```python
from build123d import *

# Parameters (mm, degrees)
SKETCH1_W           = 33
SKETCH1_H           = 37
BOSS_EXTRUDE1_DEPTH = 33
SKETCH2_R           = 13.75
CUT_EXTRUDE1_DEPTH  = 33
SKETCH3_R           = 3
CUT_EXTRUDE2_DEPTH  = 33


with BuildPart() as part:
    # Sketch1 → Boss-Extrude1 (new body)
    with BuildSketch(Plane.XY):
        with Locations((-16.5, 18.5)):
            Rectangle(SKETCH1_W, SKETCH1_H)
    extrude(amount=BOSS_EXTRUDE1_DEPTH)

    # Sketch2 → Cut-Extrude1 (cut)
    with BuildSketch(Plane.XY.offset(33)):
        with Locations((-16.5, 37)):
            Circle(SKETCH2_R)
    extrude(amount=-CUT_EXTRUDE1_DEPTH, mode=Mode.SUBTRACT)

    # Sketch3 → Cut-Extrude2 (cut)
    with BuildSketch(Plane.ZY.offset(33)):
        with Locations((16.5, 15)):
            Circle(SKETCH3_R)
    extrude(amount=-CUT_EXTRUDE2_DEPTH, mode=Mode.SUBTRACT)


solid = part.part
```
Part model, mm, in its own coordinate system. Round coordinates to 2 decimals unless told otherwise and drop trailing zeros. Order: outer loops, then holes, each group sorted by start corner. A loop starts at its lowest first (then second) coordinate and runs counter-clockwise, first axis right, second up. Notation, with made-up numbers: M 18,73 L 48,73 A17 ccw 48,106 Z; hole C -39.75,11.5 d10. An arc over 180 degrees is marked long. Put each result on its own line as item: value. Start each with the question number.
1. Drill centre lines: probe 1 along X at (y, z) = (25, 16); probe 2 along Y at (x, z) = (-24.5, 16.5); probe 3 along X at (y, z) = (32.5, 28). Where is each one in solid material? Low to high. Write a range as [from, to].
2. Slice it at B-B on y = 31. List the corners of the cut face in (x, z).
3. Drop flat-ended pins along their axis: pin 1 (3.5 mm diameter, centred on y = 15, z = 16.5, fed in from +X); pin 2 (12 mm diameter, centred on x = -18.5, z = 9.5, fed in from +Y); pin 3 (1 mm diameter, centred on x = -28, z = 14.5, fed in from +Y). Give the stop position or say it passes through.
4. Slice it at D-D on z = 10. List the corners of the cut face in (x, y), then the cut area to 3 significant figures.
5. Two-plate mould, pull along Z, no slides. Class faces 1 (the face through (-1, 37, 16)), 2 (the face through (-17, 15, 0)), 3 (the face through (-16.73, 12.07, 15.85)): +Z half, -Z half, draft (parallel to the pull), parting line (faces both ways), or undercut.
6. Slice it at A-A on x = -16.5. List the corners of the cut face in (y, z), then the cut area to 3 significant figures.
7. Slice it at C-C on z = 16.5. List the corners of the cut face in (x, y).
Findings:
1. probe 1: [-33, -23.21], [-9.79, 0]
1. probe 2: [0, 12], [18, 25.82]
1. probe 3: [-33, -29.49], [-3.51, 0]
2. outline: M -33,0 L -28.87,0 L -28.87,33 L -33,33 Z; M -4.13,0 L 0,0 L 0,33 L -4.13,33 Z
3. pin 1: through
3. pin 2: y = 25.82
3. pin 3: y = 30.29
4. outline: M -33,0 L 0,0 L 0,37 L -2.75,37 A13.75 cw -30.25,37 L -33,37 Z
4. area: 924 mm2
5. face 1: draft
5. face 2: -Z half
5. face 3: undercut
6. outline: M 0,0 L 23.25,0 L 23.25,33 L 0,33 Z; hole C 15,16.5 d6
6. area: 739 mm2
7. outline: M -33,0 L 0,0 L 0,12 L -33,12 Z; M -33,18 L 0,18 L 0,37 L -2.75,37 A13.75 cw -30.25,37 L -33,37 Z
